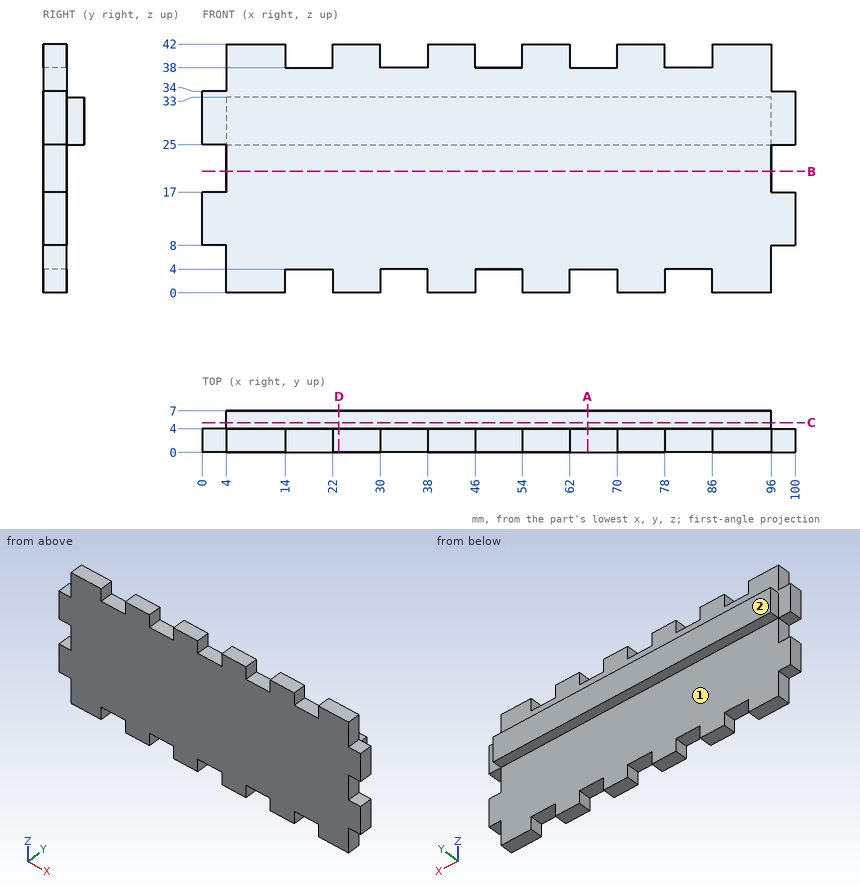
Input: dimensioned drawing with shaded views. Units: mm. Origin: part minimum x, y, z. A direction names the side the tool comes from. Give positions to 0.01 mm unless a question says otherwise; leave off trailing zeros. Write each loop counter-clockwise with the first axis right and the second up, starting at its lowest first coordinate (ties: lowest second). Pieces come first, ordered by that corner, then holes.
Q1. Section B-B, the plane z = 20.5. Output: boundary loops of the cut face in (x, y).
Q2. Section C-C, the plane y = 5. Output: boundary loops of the cut face in (x, z), plus the area to 3 significant figures.
Q3. First-contact query: P1, Ø3, axis at y = 1.5, z = 1, coming from the +X side; P2, Ø2, axis at x = 2.5, y = 2.5, coming from the -Z side; P3, Ø3, axis at y = 3.5, z = 20.5, coming from the -X side; P4, Ø1.5, axis at x = 22.5, z = 11.5, coming from the -Y side. Flat tips, straight axial feed; report the tip coordinate or a pass-through.
Q4. Section A-A, the plane x = 65. Output: boundary loops of the cut face in (y, z).
Q5. Material intervals for probe 1 along X at (y, z) = (3.25, 3.5); probe 2 along Y at (x, z) = (14, 5); probe 3 along Z at (x, y) = (76, 5), sorted ascending.
Q6. Section D-D, the plane x = 23. Output: boundary loops of the cut face in (y, z), plus the area to 3 significant figures.
Q7. Set-up query: the marked faces 1 and 2. Return all of +Z, -Z, +X, -X, +Y, -Y with unobstructed straight access to the full face (end or side cutting, diameter ignored); none if empty.
Filled in:
1. outline: (4, 0) - (96, 0) - (96, 4) - (4, 4) - close
2. outline: (4, 25) - (96, 25) - (96, 33) - (4, 33) - close
2. area: 736 mm2
3. P1: stops at x = 96
3. P2: stops at z = 8
3. P3: stops at x = 4
3. P4: stops at y = 0
4. outline: (0, 4) - (4, 4) - (4, 25) - (7, 25) - (7, 33) - (4, 33) - (4, 38) - (0, 38) - close
5. probe 1: x = 4 to 14, 22 to 30, 38 to 46, 54 to 62, 70 to 78, 86 to 96
5. probe 2: y = 0 to 4
5. probe 3: z = 25 to 33
6. outline: (0, 0) - (4, 0) - (4, 25) - (7, 25) - (7, 33) - (4, 33) - (4, 42) - (0, 42) - close
6. area: 192 mm2
7. face 1: -Z, +X, -X, +Y
7. face 2: +Z, -Z, +X, -X, +Y
